The model under review builds one solid part; all positions refer to its coordinate system, in mm. Round coordinates to 2 decimals unless told otherwise and drop trailing zeros. Write each loop counter-clockwise with the first axis right and the second up, starting at its lowest first coordinate (ties: lowest second). Pieces come first, ordered by that corner, then holes. Notation, with made-up numbers: (-4, 54) - (21, 54) arc R27 cw to (21, 78) - close; hole circle Ø3 at (76.25, 2). An arc over 180 degrees is marked (long way). One line per question, with ' | ' between items. Start each with the question number.
Autodesk Inventor part; units mm, degrees
ref_plane "YZ Plane" through (0, 0, 0) normal (1, 0, 0) x (0, 1, 0)
ref_plane "XZ Plane" through (0, 0, 0) normal (0, 1, 0) x (-1, 0, 0)
ref_plane "XY Plane" through (0, 0, 0) normal (0, 0, 1) x (1, 0, 0)
sketch "Sketch1" plane through (0, 0, 0) normal (0, 1, 0) x (-1, 0, 0)
  line L0 (0, 0) -> (93, 0)
  line L1 (93, 0) -> (93, 46.65)
  line L2 (93, 46.65) -> (0, 46.65)
  line L3 (0, 46.65) -> (0, 0)
  line L4 (74.5, 39.825) -> (18.5, 39.825) construction
  line L5 (18.5, 39.825) -> (18.5, 6.825) construction
  line L6 (18.5, 6.825) -> (74.5, 6.825) construction
  line L7 (74.5, 6.825) -> (74.5, 39.825) construction
  line L8 (74.5, 39.825) -> (93, 39.825) construction
  line L9 (74.5, 39.825) -> (74.5, 46.65) construction
  line L10 (18.5, 6.825) -> (18.5, 0) construction
  line L11 (18.5, 6.825) -> (0, 6.825) construction
  circle A0 centre (74.5, 39.825) radius 2.6
  circle A1 centre (74.5, 6.825) radius 2.6
  circle A2 centre (18.5, 6.825) radius 2.6
  circle A3 centre (18.5, 39.825) radius 2.6
  dimension "d0" = 46.65
  dimension "d1" = 93
  dimension "d2" = 33
  dimension "d3" = 56
  dimension "d4" = 5.2
  dimension "d5" = 5.2
  dimension "d6" = 5.2
  dimension "d7" = 5.2
extrude "Extrusion1" add sketch "Sketch1" along normal blind 3.5
chamfer "Chamfer1" distance 0.325 angle 45 2 edges at (-93, 1.75, 46.65) (-93, 1.75, 0)
equation "\"d5\" = d4"
equation "\"d6\" = d4"
equation "\"d7\" = d4"
properties part number "X Axis Belt Tentoner NON ADJUSTABLE Top"
1. Clearance check with a flat-ended pin moving along its axis: P1, Ø1, axis at x = -55, z = 40, coming from the -Y side. State where the tip first meets the part, or that it passes through.
2. Wall thickness on line 1 along Z through (x, y) = (-18.5, 1.25) (3 decimals); line 2 along X through (y, z) = (3.35, 7); line 3 along Z through (x, y) = (-17, 2.65): over which ranges is each line inside the solid? List them lowest first. Write a range as [from, to].
3. The part is to be moulded in two halves that separate along X. For faces 1 (the face through (-46, 0, 24)), 2 (the face through (-71.903, 1.726, 39.711)), 3 (the face through (-71.903, 1.726, 6.711)), 4 (the face through (0, 2, 24)), say which applies: pulls with the +X half, pulls with the -X half, needs draft (parallel to the pull), parting line crosses it, or undercut.
4. Add section A-A, the plane x = -74.5. Write out the cut boundary in (y, z) (3 decimals).
5. Add section B-B, the plane y = 2.65. Write out the cut boundary in (x, z) (3 decimals).
Geometry check:
1) P1: stops at y = 0
2) line 1: z = [0, 4.225], [9.425, 37.225], [42.425, 46.65] | line 2: x = [-93, -77.09], [-71.91, -21.09], [-15.91, 0] | line 3: z = [0, 4.7], [8.95, 37.7], [41.95, 46.65]
3) face 1: needs draft | face 2: undercut | face 3: undercut | face 4: pulls with the +X half
4) outline: (0, 0) - (3.5, 0) - (3.5, 4.225) - (0, 4.225) - close; (0, 9.425) - (3.5, 9.425) - (3.5, 37.225) - (0, 37.225) - close; (0, 42.425) - (3.5, 42.425) - (3.5, 46.65) - (0, 46.65) - close
5) outline: (-93, 0.325) - (-92.675, 0) - (0, 0) - (0, 46.65) - (-92.675, 46.65) - (-93, 46.325) - close; hole circle Ø5.2 at (-74.5, 6.825); hole circle Ø5.2 at (-74.5, 39.825); hole circle Ø5.2 at (-18.5, 6.825); hole circle Ø5.2 at (-18.5, 39.825)
